Build history of the part. All positions in model axes, mm. A direction names the side the tool comes from. Round coordinates to 2 decimals unless told otherwise and drop trailing zeros. Write each loop counter-clockwise with the first axis right and the second up, starting at its lowest first coordinate (ties: lowest second). Pieces come first, ordered by that corner, then holes. Notation, with made-up numbers: (42, 1) - (99, 1) arc R8 ccw to (99, 7) - close; hole circle Ø6 at (-17.5, 86.25). An arc over 180 degrees is marked (long way). Write each question's results on one line, items separated by ' | '.
from build123d import *

# Parameters (mm, degrees)
ESBO_O3_R             = 8
CORTE_EXTRUS_O2_DEPTH = 10


with BuildPart() as part:
    # Esboço1 → Revolução1 (revolve)
    with BuildSketch(Plane.XY):
        Polygon((200, 250), (300, 250), (300, 0), (0, 0), (0, 170), (200, 170), align=None)
    revolve(axis=Axis((0, 0, 0), (0, 1, 0)))

    # Esboço3 → Corte-extrusão2 (cut)
    with BuildSketch(Plane.XZ):
        with Locations((-71, 55)):
            Circle(ESBO_O3_R)
        with Locations((71, 55)):
            Circle(ESBO_O3_R)
        with Locations((71, -55)):
            Circle(ESBO_O3_R)
        with Locations((-71, -55)):
            Circle(ESBO_O3_R)
    extrude(amount=-CORTE_EXTRUS_O2_DEPTH, mode=Mode.SUBTRACT)


solid = part.part
(1) Slice it at A-A, the plane x = 0. Write the cut outline in (y, z), and give its area (3 significant figures).
Worked answers:
outline: (0, -300) - (250, -300) - (250, -200) - (170, -200) - (170, 200) - (250, 200) - (250, 300) - (0, 300) - close | area: 118,000 mm2
(2) Drill centre lines: probe 1 along Z at (x, y) = (71, 7.75); probe 2 along Y at (x, z) = (-37, -185); probe 3 along Z at (x, y) = (71, 216.5). Where is each one in solid material? Low to high. Write a range as [from, to].
Worked answers:
probe 1: z = [-291.48, -63], [-47, 47], [63, 291.48] | probe 2: y = [0, 170] | probe 3: z = [-291.48, -186.97], [186.97, 291.48]
(3) Flat gauge pins, fed straight in: pin 1 Ø2 at (x, y) = (-137, 45.5) entering from +Z; pin 2 Ø9.5 at (x, z) = (71, -55) entering from +Y; pin 3 Ø12 at (x, y) = (-222.5, 75.5) entering from +Z. Where does each tip first touch, or does it go through?
Worked answers:
pin 1: stops at z = 267.4 | pin 2: stops at y = 170 | pin 3: stops at z = 207.67
(4) Slice it at C-C, the plane z = 0. Write the cut outline in (x, y), and give its area (3 significant figures).
Worked answers:
outline: (-300, 0) - (300, 0) - (300, 250) - (200, 250) - (200, 170) - (-200, 170) - (-200, 250) - (-300, 250) - close | area: 118,000 mm2
(5) Tool access for faces 4 (the flat face through (-4, 0, -4)), 5 (the cylindrical face through (190.764, 210.56, -60.075)), 6 (the cylindrical face through (65.1, 4.9, 60.4)): list every direction of +Z, -Z, +X, -X, +Y, -Y with a clear straight run to the whole face (end or side of a thin tool).
Worked answers:
face 4: +Z, -Z, +X, -X, -Y | face 5: +Y | face 6: -Y
(6) Slice it at D-D, the plane x = -71. Write the cut outline in (y, z), and give its area (3 significant figures).
Worked answers:
outline: (0, -291.48) - (250, -291.48) - (250, -186.97) - (170, -186.97) - (170, 186.97) - (250, 186.97) - (250, 291.48) - (0, 291.48) - (0, 63) - (10, 63) - (10, 47) - (0, 47) - (0, -47) - (10, -47) - (10, -63) - (0, -63) - close | area: 116,000 mm2
(7) Slice it at B-B, the plane y = 179.5. Write the cut outline in (x, z).
Worked answers:
outline: circle Ø600 at (0, 0); hole circle Ø400 at (0, 0)
(8) Two-plate mould, pull along Z, no slides. Class faces 1 (the flat face through (-71, 10, 55)), 2 (the cylindrical face through (-39.054, 123.25, -297.447)), 3 (the flat face through (-196, 250, 62)): released by +Z, released by -Z, zero draft, split by the parting line, or undercut.
Worked answers:
face 1: undercut | face 2: split by the parting line | face 3: zero draft
